from build123d import *

# Parameters (mm, degrees)
F0_W     = 2
F0_H     = 6.473958
F1_DEPTH = 28.3
F2_W     = 2
F2_H     = 8
F3_DEPTH = 12
F4_W     = 2
F4_H     = 4.3
F5_DEPTH = 35
F6_W     = 2
F6_H     = 8.3
F7_DEPTH = 25


with BuildPart() as f1:
    # F0 (on Top) → F1 (new body)
    with BuildSketch(Plane.XY):
        Polygon((55.053259, 41.889014), (0.053259, 41.889014), (0.053259, 37.194386), (2.053259, 37.194386), (2.053259, 39.889014), (48.263833, 39.889014), (48.263833, 38.826488), (53.053259, 38.826488), (53.053259, 1.889014), (51.531006, 1.889014), (51.531006, -0.110986), (55.053259, -0.110986), align=None)
        Polygon((0.053259, 6.720428), (0.053259, -0.110986), (42.531006, -0.110986), (42.531006, 1.889014), (2.053259, 1.889014), (2.053259, 6.720428), align=None)
        with Locations((1.053259, 21.957407)):
            Rectangle(F0_W, F0_H)
    extrude(amount=F1_DEPTH)

    # F2 (on face) → F3 (join)
    with BuildSketch(Plane.XZ.offset(-37.194386)):
        with Locations((1.053259, 4)):
            Rectangle(F2_W, F2_H)
    extrude(amount=F3_DEPTH)

    # F4 (on face) → F5 (join)
    with BuildSketch(Plane.XZ.offset(-37.194386)):
        with Locations((1.053259, 26.15)):
            Rectangle(F4_W, F4_H)
    extrude(amount=F5_DEPTH)

    # F6 (on face) → F7 (join)
    with BuildSketch(Plane(origin=(51.531006, 0, 0), x_dir=(0, -1, 0), z_dir=(-1, 0, 0))):
        with Locations((-0.889014, 24.15)):
            Rectangle(F6_W, F6_H)
    extrude(amount=F7_DEPTH)


solid = f1.part
Can you work these out from the model? Positions are in its coordinate system, mm. A direction names the side the tool comes from. Round coordinates to 2 decimals unless told otherwise and drop trailing zeros. Write each loop counter-clockwise with the first axis right and the second up, starting at its lowest first coordinate (ties: lowest second). Pieces come first, ordered by that corner, then holes. Notation, with made-up numbers: (69, 25.25) -> (88, 25.25) arc R25 ccw to (88, 52.25) -> close; hole circle Ø2 at (85, -3). An arc over 180 degrees is marked (long way). One line per question, with ' | ' between items. Start each with the question number.
1) I need wall thicknesses on line 1 (Y direction, x = 29, z = 12); line 2 (X direction, y = 8, z = 24.5); line 3 (X direction, y = 31, z = 11.5). Which ranges of each line are inside material? Lowest first, please. Write a range as [from, to].
2) Suppose I cut it at C-C on z = 17.5. Write out the boundary of the cut face in (x, y), then the cut area to 3 significant figures.
3) Suppose I cut it at D-D on y = 20. Write out the boundary of the cut face in (x, z), then the cut area to 3 significant figures.
4) I'm going to push flat-ended pins straight in: P1, Ø0.6, axis at x = 1.5, y = 29, coming from the -Z side; P2, Ø2, axis at x = 47, y = 0.5, coming from the -Z side; P3, Ø1.6, axis at x = 1.5, y = 13.5, coming from the -Z side. Where does each tip first touch, or does it pass through?
5) Suppose I cut it at B-B on x = 41.5. Write out the boundary of the cut face in (y, z).
6) Suppose I cut it at A-A on y = 34. Write out the boundary of the cut face in (x, z), then the cut area to 3 significant figures.
7) If we mould it in two halves opening along Z, with no side actions, what happens to faces 5 (the flat face through (1, 6.72, 12)), 6 (the flat face through (47, 1, 20)), 7 (the flat face through (1, 31, 24))? For each: released by +Z, released by -Z, zero draft, split by the parting line, or undercut.
8) On a 3-axis mill with a long thin cutter (end or side, diameter ignored), from which of +Z, -Z, +X, -X, +Y, -Y can I reach the whole of each face in a straight line? I mean faces 1 (the flat face through (1, 37.194, 16)), 2 (the flat face through (42.531, 1, 10)), 3 (the flat face through (51, 38.826, 14)), 4 (the flat face through (1, 13, 24)). Say none if no direction works.
Return value:
1) line 1: y = [-0.11, 1.89], [39.89, 41.89] | line 2: x = [0.05, 2.05], [53.05, 55.05] | line 3: x = [53.05, 55.05]
2) outline: (0.05, -0.11) -> (42.53, -0.11) -> (42.53, 1.89) -> (2.05, 1.89) -> (2.05, 6.72) -> (0.05, 6.72) -> close; (0.05, 18.72) -> (2.05, 18.72) -> (2.05, 25.19) -> (0.05, 25.19) -> close; (0.05, 37.19) -> (2.05, 37.19) -> (2.05, 39.89) -> (48.26, 39.89) -> (48.26, 38.83) -> (53.05, 38.83) -> (53.05, 1.89) -> (51.53, 1.89) -> (51.53, -0.11) -> (55.05, -0.11) -> (55.05, 41.89) -> (0.05, 41.89) -> close | area: 311 mm2
3) outline: (0.05, 0) -> (2.05, 0) -> (2.05, 28.3) -> (0.05, 28.3) -> close; (53.05, 0) -> (55.05, 0) -> (55.05, 28.3) -> (53.05, 28.3) -> close | area: 113 mm2
4) P1: stops at z = 0 | P2: stops at z = 20 | P3: stops at z = 24
5) outline: (-0.11, 0) -> (1.89, 0) -> (1.89, 28.3) -> (-0.11, 28.3) -> close; (39.89, 0) -> (41.89, 0) -> (41.89, 28.3) -> (39.89, 28.3) -> close
6) outline: (0.05, 0) -> (2.05, 0) -> (2.05, 8) -> (0.05, 8) -> close; (0.05, 24) -> (2.05, 24) -> (2.05, 28.3) -> (0.05, 28.3) -> close; (53.05, 0) -> (55.05, 0) -> (55.05, 28.3) -> (53.05, 28.3) -> close | area: 81.2 mm2
7) face 5: zero draft | face 6: released by -Z | face 7: undercut
8) face 1: -X | face 2: -Z, -Y | face 3: +Z, -Z | face 4: -Z, -X
